from build123d import *

# Parameters (mm, degrees)
BOSS_EXTRUDE1_DEPTH = 350
FILLET1_R           = 5
SKETCH2_R           = 5
CUT_EXTRUDE1_DEPTH  = 300
SKETCH3_R           = 5
SKETCH3_W           = 30
SKETCH3_H           = 70
CUT_EXTRUDE6_DEPTH  = 10


with BuildPart() as part:
    # Sketch1 → Boss-Extrude1 (new body)
    with BuildSketch(Plane.XY):
        Polygon((0, 0), (200, 0), (200, 30), (196, 30), (196, 4), (4, 4), (4, 30), (0, 30), align=None)
    extrude(amount=BOSS_EXTRUDE1_DEPTH)

    # Fillet1
    fillet1_edges = [part.edges().sort_by_distance(p)[0] for p in [
        (4, 4, 175),
        (196, 4, 175),
        (200, 0, 175),
        (0, 0, 175),
    ]]
    fillet(fillet1_edges, radius=FILLET1_R)

    # Sketch2 → Cut-Extrude1 (cut)
    with BuildSketch(Plane(origin=(200, 0, 0), x_dir=(0, 0, -1), z_dir=(1, 0, 0))):
        with Locations((-315, 17)):
            Circle(SKETCH2_R)
        with Locations((-35, 17)):
            Circle(SKETCH2_R)
    extrude(amount=-CUT_EXTRUDE1_DEPTH, mode=Mode.SUBTRACT)

    # Sketch3 → Cut-Extrude6 (cut)
    with BuildSketch(Plane(origin=(0, 0, 0), x_dir=(1, 0, 0), z_dir=(0, 1, 0))):
        with Locations((30.894933586, -54.066133776)):
            Circle(SKETCH3_R)
        with Locations((169.105066414, -54.066133776)):
            Circle(SKETCH3_R)
        with Locations((169.105066414, -295.933866224)):
            Circle(SKETCH3_R)
        with Locations((30.894933586, -295.933866224)):
            Circle(SKETCH3_R)
        with Locations((100, -175)):
            Rectangle(SKETCH3_W, SKETCH3_H)
    extrude(amount=CUT_EXTRUDE6_DEPTH, mode=Mode.SUBTRACT)


solid = part.part
Verification items for the finished model (mm, model axes). A direction names the side the tool comes from. Give positions to 0.01 mm unless a question says otherwise; leave off trailing zeros. Loops run counter-clockwise (first coordinate to the right, second up) from the corner with the lowest first, then second, coordinate; pieces in that order, holes last.
1. Cross-section at D-D on z = 315. Record the cut outline in (x, y), and give its area (3 significant figures).
Derived:
outline: (0, 5) arc R5 ccw to (5, 0) - (195, 0) arc R5 ccw to (200, 5) - (200, 12) - (196, 12) - (196, 9) arc R5 cw to (191, 4) - (9, 4) arc R5 cw to (4, 9) - (4, 12) - (0, 12) - close; (0, 22) - (4, 22) - (4, 30) - (0, 30) - close; (196, 22) - (200, 22) - (200, 30) - (196, 30) - close
area: 928 mm2
2. Release check for a two-part mould opening along X. For faces 3 (the flat face through (85, 2, 0)), 4 (the flat face through (0, 18, 173)), 5 (the cylindrical face through (33.583, 1.972, 291.718)) record: +X half, -X half, draft (parallel to the pull), parting line (faces both ways), or undercut.
Derived:
face 3: draft
face 4: -X half
face 5: undercut
3. Cross-section at A-A on y = 17. Record the cut outline in (x, z).
Derived:
outline: (0, 0) - (4, 0) - (4, 30) - (0, 30) - close; (0, 40) - (4, 40) - (4, 310) - (0, 310) - close; (0, 320) - (4, 320) - (4, 350) - (0, 350) - close; (196, 0) - (200, 0) - (200, 30) - (196, 30) - close; (196, 40) - (200, 40) - (200, 310) - (196, 310) - close; (196, 320) - (200, 320) - (200, 350) - (196, 350) - close
4. Tool access check on faces 1 (the cylindrical face through (173.874, 1.972, 52.564)), 2 (the flat face through (196, 20, 173)). Record the directions out of +Z, -Z, +X, -X, +Y, -Y that give a thin tool (end or side, any length) a straight path to the whole face; none if there is none.
Derived:
face 1: +Y, -Y
face 2: +Z, -Z, +Y
5. Go/stop test with flat-tipped pins: P1, Ø1.2, axis at y = 1, z = 161, coming from the +X side; P2, Ø10, axis at x = 30.5, z = 53.5, coming from the +Y side; P3, Ø2, axis at y = 2, z = 176.5, coming from the -X side. Record where each tip stops, or that it passes through.
Derived:
P1: stops at x = 198.67
P2: stops at y = 4
P3: stops at x = 0.42
6. Material ranges on probe 1 along X at (y, z) = (15.25, 198); probe 2 along Y at (x, z) = (19, 58.5); probe 3 along Y at (x, z) = (198.6, 315), recorded low to high.
Derived:
probe 1: x = 0 to 4, 196 to 200
probe 2: y = 0 to 4
probe 3: y = 1.53 to 12, 22 to 30
7. Cross-section at B-B on z = 153.5. Record the cut outline in (x, y), and give its area (3 significant figures).
Derived:
outline: (0, 5) arc R5 ccw to (5, 0) - (85, 0) - (85, 4) - (9, 4) arc R5 cw to (4, 9) - (4, 30) - (0, 30) - close; (115, 0) - (195, 0) arc R5 ccw to (200, 5) - (200, 30) - (196, 30) - (196, 9) arc R5 cw to (191, 4) - (115, 4) - close
area: 888 mm2
8. Cross-section at C-C on x = 101. Record the cut outline in (y, z).
Derived:
outline: (0, 0) - (4, 0) - (4, 140) - (0, 140) - close; (0, 210) - (4, 210) - (4, 350) - (0, 350) - close
